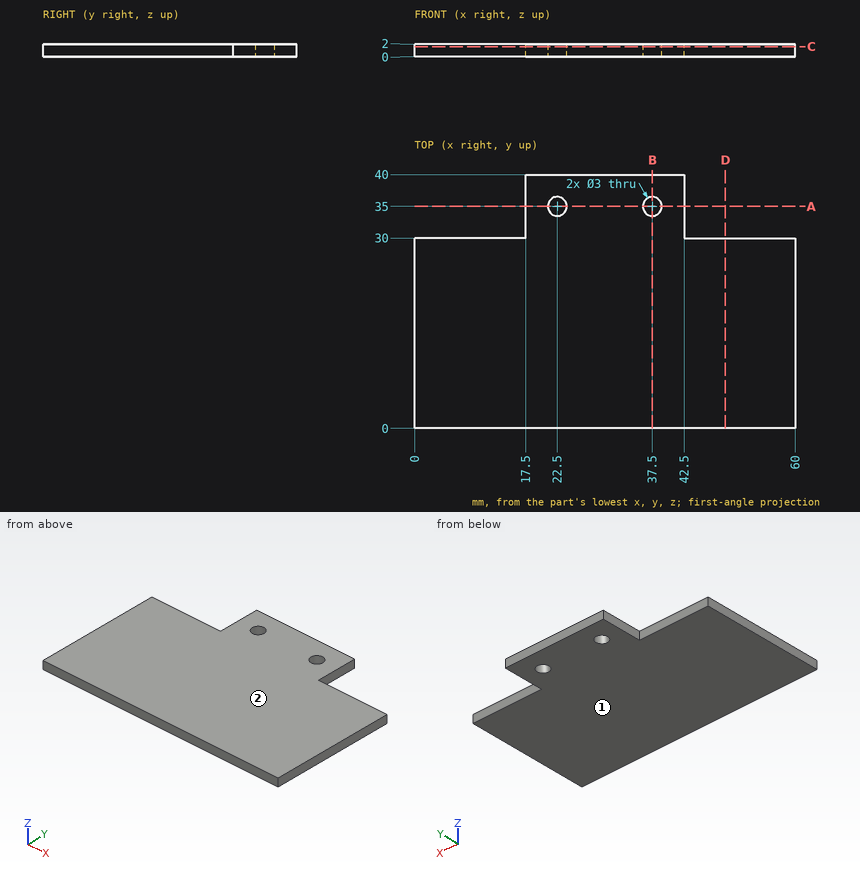
Geometry: see drawing. Coordinates: mm, zero at the bounding-box minimum. Coordinates: 2 decimals unless noted, no trailing zeros. Loops run counter-clockwise (first coordinate to the right, second up) from the corner with the lowest first, then second, coordinate; pieces in that order, holes last. Notation, with made-up numbers: (-15, -16) - (18, -16) arc R24 cw to (18, -3) - close; hole circle Ø6 at (85.25, 61). An arc over 180 degrees is marked (long way). Return JSON: item names as keys, results as strings.
Q1. Section C-C, the plane z = 1.6. Return loops of the section in (x, y).
Results:
{"outline": "(0, 0) - (60, 0) - (60, 30) - (42.5, 30) - (42.5, 40) - (17.5, 40) - (17.5, 30) - (0, 30) - close; hole circle Ø3 at (22.5, 35); hole circle Ø3 at (37.5, 35)"}
Q2. Section B-B, the plane x = 37.5. Return loops of the section in (y, z), plus the area to 3 significant figures.
Results:
{"outline": "(0, 0) - (33.5, 0) - (33.5, 2) - (0, 2) - close; (36.5, 0) - (40, 0) - (40, 2) - (36.5, 2) - close", "area": "74.0 mm2"}
Q3. Material intervals for line 1 along Y through (x, z) = (37.5, 0.7); line 2 along Y through (x, z) = (12.5, 1.9); line 3 along X through (y, z) = (37, 1.85), sorted ascending.
Results:
{"line 1": "0 to 33.5, 36.5 to 40", "line 2": "0 to 30", "line 3": "17.5 to 42.5"}
Q4. Contact query for flat-ended pins moving along their axis: P1, Ø0.6, axis at y = 37, z = 1, coming from the -X side; P2, Ø1, axis at y = 35.5, z = 1.5, coming from the +X side; P3, Ø2.5, axis at x = 37.5, y = 35, coming from the +Z side. Output: stop coordinate, or through.
Results:
{"P1": "x = 17.5", "P2": "x = 42.5", "P3": "through"}
Q5. Mould query, pull axis Z, two halves, no side actions, for the marked faces 1 and 2. Classes: released by +Z, released by -Z, zero draft, split by the parting line, or undercut.
Results:
{"face 1": "released by -Z", "face 2": "released by +Z"}
Q6. Section D-D, the plane x = 49. Return loops of the section in (y, z), plus the area to 3 significant figures.
Results:
{"outline": "(0, 0) - (30, 0) - (30, 2) - (0, 2) - close", "area": "60.0 mm2"}
Q7. Section A-A, the plane y = 35. Return loops of the section in (x, z).
Results:
{"outline": "(17.5, 0) - (21, 0) - (21, 2) - (17.5, 2) - close; (24, 0) - (36, 0) - (36, 2) - (24, 2) - close; (39, 0) - (42.5, 0) - (42.5, 2) - (39, 2) - close"}
